Geometry: final body of the model. Coordinates: model frame, mm. A direction names the side the tool comes from. Give positions to 0.01 mm unless a question says otherwise; leave off trailing zeros. Write each loop counter-clockwise with the first axis right and the second up, starting at its lowest first coordinate (ties: lowest second). Pieces come first, ordered by that corner, then holes.
from build123d import *

# Parameters (mm, degrees)
SKETCH1_W           = 23
SKETCH1_H           = 12.1
BOSS_EXTRUDE1_DEPTH = 23.2
SKETCH2_W           = 12.1
SKETCH2_H           = 2.3
BOSS_EXTRUDE2_DEPTH = 4.75
SKETCH3_R           = 1
CUT_EXTRUDE1_DEPTH  = 2.3
SKETCH4_R           = 6.05
BOSS_EXTRUDE3_DEPTH = 4
SKETCH5_R           = 3.575
BOSS_EXTRUDE4_DEPTH = 4.75
BOSS_EXTRUDE5_DEPTH = 1.6


with BuildPart() as part:
    # Sketch1 → Boss-Extrude1 (new body)
    with BuildSketch(Plane(origin=(0, 0, 0), x_dir=(1, 0, 0), z_dir=(0, 1, 0))):
        Rectangle(SKETCH1_W, SKETCH1_H)
    extrude(amount=BOSS_EXTRUDE1_DEPTH)

    # Sketch2 → Boss-Extrude2 (add)
    with BuildSketch(Plane(origin=(11.5, 0, 0), x_dir=(0, 0, -1), z_dir=(1, 0, 0))):
        with Locations((0, 17.35)):
            Rectangle(SKETCH2_W, SKETCH2_H)
    boss_extrude2 = extrude(amount=BOSS_EXTRUDE2_DEPTH)

    # Sketch3 → Cut-Extrude1 (cut)
    with BuildSketch(Plane(origin=(0, 18.5, 0), x_dir=(1, 0, 0), z_dir=(0, 1, 0))):
        with Locations((13.8, 0)):
            Circle(SKETCH3_R)
    cut_extrude1 = extrude(amount=-CUT_EXTRUDE1_DEPTH, mode=Mode.SUBTRACT)

    # Mirror1: Boss-Extrude2, Cut-Extrude1 across plane
    add(boss_extrude2.mirror(Plane(origin=(0, 0, 0), x_dir=(0, 0, 1), z_dir=(1, 0, 0))))
    add(cut_extrude1.mirror(Plane(origin=(0, 0, 0), x_dir=(0, 0, 1), z_dir=(1, 0, 0))), mode=Mode.SUBTRACT)

    # Sketch4 → Boss-Extrude3 (add)
    with BuildSketch(Plane(origin=(0, 23.2, 0), x_dir=(1, 0, 0), z_dir=(0, 1, 0))):
        with Locations((-5.45, 0)):
            Circle(SKETCH4_R)
    extrude(amount=BOSS_EXTRUDE3_DEPTH)

    # Sketch5 → Boss-Extrude4 (add)
    with BuildSketch(Plane(origin=(0, 27.2, 0), x_dir=(1, 0, 0), z_dir=(0, 1, 0))):
        with Locations((-5.45, 0)):
            Circle(SKETCH5_R)
    extrude(amount=BOSS_EXTRUDE4_DEPTH)

    # Sketch7 → Boss-Extrude5 (add)
    with BuildSketch(Plane(origin=(0, 31.95, 0), x_dir=(1, 0, 0), z_dir=(0, 1, 0))):
        with BuildLine():
            Line((10.55, 2), (-4.752926477, 3.506381825))
            ThreePointArc((-4.752926477, 3.506381825), (-2.68660871, 2.26810352), (-1.875, 0))
            ThreePointArc((-1.875, 0), (-2.68660871, -2.26810352), (-4.752926477, -3.506381825))
            Line((-4.752926477, -3.506381825), (10.55, -2))
            ThreePointArc((10.55, -2), (12.55, 0), (10.55, 2))
        make_face()
    extrude(amount=-BOSS_EXTRUDE5_DEPTH)


solid = part.part
Q1. Ray query, line 1 along X through (y, z) = (17.85, 0); line 2 along Z through (x, y) = (13.8, 17.8); line 3 along Y through (x, z) = (0, 1). Return the intervals inside material, ascending.
Filled sheet:
line 1: x = -16.25 to -14.8, -12.8 to 12.8, 14.8 to 16.25
line 2: z = -6.05 to -1, 1 to 6.05
line 3: y = 0 to 27.2, 30.35 to 31.95
Q2. Section D-D on x = 8. Output: boundary loops of the cut face in (y, z).
Filled sheet:
outline: (0, -6.05) - (23.2, -6.05) - (23.2, 6.05) - (0, 6.05) - close; (30.35, -2.25) - (31.95, -2.25) - (31.95, 2.25) - (30.35, 2.25) - close
Q3. Pull-direction query (X, two-part tool) for faces 6 (the flat face through (11.5, 8, 0)), 7 (the flat face through (-11.5, 21, 0)), 8 (the flat face through (15, 16.2, 0)), 9 (the cylindrical face through (14.754, 17.366, -0.3)); classes: released by +X, released by -X, zero draft, split by the parting line, or undercut.
Filled sheet:
face 6: released by +X
face 7: released by -X
face 8: zero draft
face 9: undercut
Q4. Section C-C on y = 21.5. Output: boundary loops of the cut face in (x, z).
Filled sheet:
outline: (-11.5, -6.05) - (11.5, -6.05) - (11.5, 6.05) - (-11.5, 6.05) - close
Q5. Section A-A on x = 13.8. Output: boundary loops of the cut face in (y, z).
Filled sheet:
outline: (16.2, -6.05) - (18.5, -6.05) - (18.5, -1) - (16.2, -1) - close; (16.2, 1) - (18.5, 1) - (18.5, 6.05) - (16.2, 6.05) - close
Q6. Section B-B on z = 2.75. Output: boundary loops of the cut face in (x, y), plus the area to 3 significant figures.
Filled sheet:
outline: (-16.25, 16.2) - (-11.5, 16.2) - (-11.5, 0) - (11.5, 0) - (11.5, 16.2) - (16.25, 16.2) - (16.25, 18.5) - (11.5, 18.5) - (11.5, 23.2) - (-0.06, 23.2) - (-0.06, 27.2) - (-3.17, 27.2) - (-3.17, 30.35) - (2.93, 30.35) - (2.93, 31.95) - (-7.73, 31.95) - (-7.73, 27.2) - (-10.84, 27.2) - (-10.84, 23.2) - (-11.5, 23.2) - (-11.5, 18.5) - (-16.25, 18.5) - close
area: 630 mm2
Q7. Access query for faces 1 (the flat face through (11.5, 21, 0)), 2 (the flat face through (-10, 23.2, 5)), 3 (the flat face through (2.791, 31.161, 2.764)), 4 (the cylindrical face through (-9.02, 29.01, -0.16)), 5 (the flat face through (-15, 16.2, 0)). Directions: +Z, -Z, +X, -X, +Y, -Y. A direction counts if a zero-diameter tool reaches every point of the face in a straight line with its end or side. Return the directions, or none.
Filled sheet:
face 1: +Z, -Z, +X
face 2: +Z, -X, +Y
face 3: +Z, +X, +Y
face 4: none
face 5: +Z, -Z, -X, -Y
Q8. Pin query (flat end, axial travel): P1, Ø2.5, axis at y = 22, z = -2, coming from the -X side; P2, Ø3, axis at x = -10, z = 4, coming from the +Y side; P3, Ø6, axis at y = 10, z = -0.5, coming from the +X side. Return the tip coordinate at first contact, or that it passes through.
Filled sheet:
P1: stops at x = -11.5
P2: stops at y = 27.2
P3: stops at x = 11.5
